Geometry check sheet. Reference: the model listing, model coordinates, mm. A direction names the side the tool comes from. Coordinates: 2 decimals unless noted, no trailing zeros. Order: outer loops, then holes, each group sorted by start corner. A loop starts at its lowest first (then second) coordinate and runs counter-clockwise, first axis right, second up. Notation, with made-up numbers: (48.5, -22) - (101.5, -22) arc R18 cw to (101.5, 13) - close; hole circle Ø4 at (75, -13.5). An arc over 180 degrees is marked (long way). Use CSV: the item, a comma, the result in double quotes. Start each with the question number.
1) Draft check along Z on faces 1 (the flat face through (-4, 0, 5)), 2 (the flat face through (-31, -13, -45.608)), 3 (the cylindrical face through (4.081, -12.522, 50.538)), 4 (the cylindrical face through (-51.136, -12.522, -57.326)). Enter one of: released by +Z, released by -Z, zero draft, split by the parting line, or undercut.
2) Thickness scan on probe 1 along Z at (x, y) = (-35, -23.25); probe 2 along Z at (x, y) = (3.5, -15.25); probe 3 along Z at (x, y) = (-44, -16.5). Record the ranges inside material, lowest first. Write a range as [from, to].
3) Tool access check on faces 5 (the cylindrical face through (-14.022, -12.522, -42.907)), 6 (the flat face through (12.5, -12.5, -29)). Record the directions out of +Z, -Z, +X, -X, +Y, -Y that give a thin tool (end or side, any length) a straight path to the whole face; none if there is none.
4) Sectioned sample at A-A, the plane y = -17.5. Count the separate pieces of the cut face and the enclosed holes in it, and give its area (3 significant figures).
5) Depth check by flat-ended pin: P1, Ø3, axis at y = -22.5, z = -36, coming from the +X side; P2, Ø10, axis at x = -24, z = -19, coming from the -Y side; P3, Ø8, axis at y = -8.5, z = 9, coming from the +X side; P4, Ø12, axis at x = -27.5, y = -10, coming from the -Z side. Enter the tip coordinate at first touch or a pass-through.
6) Sectioned sample at C-C, the plane x = -25. Record the cut outline in (y, z).
7) Sectioned sample at B-B, the plane z = 41. Record the cut outline in (x, y), and give its area (3 significant figures).
from build123d import *

# Parameters (mm, degrees)
F0_R     = 2.8919986146
F1_DEPTH = 25.4


with BuildPart() as f1:
    # F0 (on Front) → F1 (new body)
    with BuildSketch(Plane.XZ):
        with BuildLine():
            ThreePointArc((-15.7877418604, -1.6621768702), (-15.875, -1.428e-07), (-15.7877418904, 1.6621765861))
            Line((-15.7877418904, 1.6621765861), (-15.9627403992, 0))
            Line((-15.9627403992, 0), (-15.7877418604, -1.6621768702))
        make_face()
        with BuildLine():
            ThreePointArc((15.6388934197, -2.7277532162), (15.7630306925, -1.8821499378), (15.8414795915, -1.0310913397))
            Line((15.8414795915, -1.0310913397), (15.6388934197, -2.7277532162))
        make_face()
        with BuildLine():
            ThreePointArc((15.7859080775, 1.6795032503), (15.8527113727, 0.8409323008), (15.875, 0))
            ThreePointArc((15.875, 0), (15.8666176849, -0.515818032), (15.8414795915, -1.0310913397))
            Line((15.8414795915, -1.0310913397), (15.9645947804, 0))
            Line((15.9645947804, 0), (15.7859080775, 1.6795032503))
        make_face()
        with BuildLine():
            ThreePointArc((0, -62.890048396), (6.3233352792, -60.4883240433), (9.4578184155, -54.4943383586))
            ThreePointArc((9.4578184155, -54.4943383586), (9.5081897701, -53.9306916548), (9.525, -53.365048396))
            ThreePointArc((9.525, -53.365048396), (6.7351920908, -46.6298563052), (0, -43.840048396))
            Line((0, -43.840048396), (0, -50.190048396))
            ThreePointArc((0, -50.190048396), (2.2450640303, -51.1199843657), (3.175, -53.365048396))
            ThreePointArc((3.175, -53.365048396), (-0.0112439351, -56.5400284863), (-3.1749203615, -53.3425606669))
            Line((-3.1749203615, -53.3425606669), (-9.5247610846, -53.2975852086))
            ThreePointArc((-9.5247610846, -53.2975852086), (-7.0387492113, -59.7823402345), (-0.8107396043, -62.8554818052))
            Line((-0.8107396043, -62.8554818052), (0, -62.890048396))
        make_face()
        with BuildLine():
            ThreePointArc((-41.6894964213, -45.607795813), (-50.980516261, -57.5603975821), (-36.5115841576, -53.1064395112))
            ThreePointArc((-36.5115841576, -53.1064395112), (-36.5114348356, -53.078330026), (-36.5113850614, -53.0502201884))
            ThreePointArc((-36.5113850614, -53.0502201884), (-37.9332671482, -48.5169399787), (-41.6894964213, -45.607795813))
        make_face()
        with BuildLine():
            ThreePointArc((-41.7578870296, -53.0502201884), (-41.7579039042, -53.0597500804), (-41.7579545278, -53.0692798529))
            ThreePointArc((-41.7579545278, -53.0692798529), (-47.1398662186, -53.0406902964), (-41.7578870296, -53.0502201884))
        make_face(mode=Mode.SUBTRACT)
        with BuildLine():
            ThreePointArc((-15.7877418904, 1.6621765861), (-10.6214069618, 11.7983617147), (0, 15.875))
            Line((0, 15.875), (0, 51.409951604))
            ThreePointArc((0, 51.409951604), (-6.8199440232, 54.2855915957), (-9.5219449967, 61.1761744869))
            Line((-9.5219449967, 61.1761744869), (-15.7877418904, 1.6621765861))
        make_face()
        with BuildLine():
            Line((9.4578184155, -54.4943383586), (15.6388934197, -2.7277532162))
            ThreePointArc((15.6388934197, -2.7277532162), (10.215491733, -12.1515165166), (0, -15.875))
            Line((0, -15.875), (0, -43.840048396))
            ThreePointArc((0, -43.840048396), (6.7351920908, -46.6298563052), (9.525, -53.365048396))
            ThreePointArc((9.525, -53.365048396), (9.5081897701, -53.9306916548), (9.4578184155, -54.4943383586))
        make_face()
        with BuildLine():
            ThreePointArc((0, 51.409951604), (6.6108879801, 54.077708345), (9.5186282495, 60.5866108977))
            ThreePointArc((9.5186282495, 60.5866108977), (9.5234069292, 60.7607521157), (9.525, 60.934951604))
            ThreePointArc((9.525, 60.934951604), (0.1206211137, 70.4591878226), (-9.5219449967, 61.1761744869))
            ThreePointArc((-9.5219449967, 61.1761744869), (-6.8199440232, 54.2855915957), (0, 51.409951604))
        make_face()
        with BuildLine():
            ThreePointArc((3.175, 60.934951604), (2.2450640303, 58.6898875738), (0, 57.759951604))
            ThreePointArc((0, 57.759951604), (-2.2450640303, 63.1800156343), (3.175, 60.934951604))
        make_face(mode=Mode.SUBTRACT)
        with BuildLine():
            Line((0, -50.190048396), (0, -43.840048396))
            ThreePointArc((0, -43.840048396), (-6.7112978678, -46.6060465518), (-9.5247610846, -53.2975852086))
            Line((-9.5247610846, -53.2975852086), (-3.1749203615, -53.3425606669))
            ThreePointArc((-3.1749203615, -53.3425606669), (-2.2370992893, -51.1120477812), (0, -50.190048396))
        make_face()
        with BuildLine():
            ThreePointArc((0, 15.875), (10.6149307794, 11.8041886443), (15.7859080775, 1.6795032503))
            Line((15.7859080775, 1.6795032503), (9.5186282495, 60.5866108977))
            ThreePointArc((9.5186282495, 60.5866108977), (6.6108879801, 54.077708345), (0, 51.409951604))
            Line((0, 51.409951604), (0, 15.875))
        make_face()
        with Locations((4.4577782974, 47.6701632142)):
            Circle(F0_R, mode=Mode.SUBTRACT)
        with BuildLine():
            Line((0, -43.840048396), (0, -15.875))
            ThreePointArc((0, -15.875), (-10.6214068556, -11.7983618103), (-15.7877418604, -1.6621768702))
            Line((-15.7877418604, -1.6621768702), (-12.0856847125, -36.8251776935))
            ThreePointArc((-12.0856847125, -36.8251776935), (-14.0835662669, -42.9767963876), (-19.9921858423, -45.607795813))
            Line((-19.9921858423, -45.607795813), (-41.6894964213, -45.607795813))
            ThreePointArc((-41.6894964213, -45.607795813), (-37.9332671482, -48.5169399787), (-36.5113850614, -53.0502201884))
            ThreePointArc((-36.5113850614, -53.0502201884), (-36.5114348356, -53.078330026), (-36.5115841576, -53.1064395112))
            Line((-36.5115841576, -53.1064395112), (-9.5247610846, -53.2975852086))
            ThreePointArc((-9.5247610846, -53.2975852086), (-6.7112978678, -46.6060465518), (0, -43.840048396))
        make_face()
        with BuildLine():
            Line((0, 3.175), (0, 15.875))
            ThreePointArc((0, 15.875), (-10.6214069618, 11.7983617147), (-15.7877418904, 1.6621765861))
            ThreePointArc((-15.7877418904, 1.6621765861), (-15.875, -1.428e-07), (-15.7877418604, -1.6621768702))
            ThreePointArc((-15.7877418604, -1.6621768702), (-10.6214068556, -11.7983618103), (0, -15.875))
            Line((0, -15.875), (0, -3.175))
            ThreePointArc((0, -3.175), (-3.175, 0), (0, 3.175))
        make_face()
        with BuildLine():
            ThreePointArc((15.8414795915, -1.0310913397), (15.8666176849, -0.515818032), (15.875, 0))
            ThreePointArc((15.875, 0), (15.8527113727, 0.8409323008), (15.7859080775, 1.6795032503))
            ThreePointArc((15.7859080775, 1.6795032503), (10.6149307794, 11.8041886443), (0, 15.875))
            Line((0, 15.875), (0, 3.175))
            ThreePointArc((0, 3.175), (2.2450640303, 2.2450640303), (3.175, 0))
            ThreePointArc((3.175, 0), (2.2450640303, -2.2450640303), (0, -3.175))
            Line((0, -3.175), (0, -15.875))
            ThreePointArc((0, -15.875), (10.215491733, -12.1515165166), (15.6388934197, -2.7277532162))
            Line((15.6388934197, -2.7277532162), (15.8414795915, -1.0310913397))
        make_face()
        with BuildLine():
            ThreePointArc((-0.8107396043, -62.8554818052), (-0.405738079, -62.8814028246), (0, -62.890048396))
            Line((0, -62.890048396), (-0.8107396043, -62.8554818052))
        make_face()
    extrude(amount=F1_DEPTH)


solid = f1.part
Evaluation:
1,face 1,"zero draft"
1,face 2,"released by +Z"
1,face 3,"undercut"
1,face 4,"split by the parting line"
2,probe 1,"[-53.12, -45.61]"
2,probe 2,"[-62.22, 44.94], [50.4, 69.79]"
2,probe 3,"[-60.98, -55.7], [-50.4, -45.13]"
3,face 5,"+Y, -Y"
3,face 6,"-Z, +X, +Y, -Y"
4,separate pieces,"1"
4,enclosed holes,"5"
4,area,"3,500 mm²"
5,P1,"x = 11.85"
5,P2,"through"
5,P3,"x = 15.43"
5,P4,"z = -53.21"
6,outline,"(-25.4, -53.19) - (0, -53.19) - (0, -45.61) - (-25.4, -45.61) - close"
7,outline,"(-11.65, -25.4) - (11.6, -25.4) - (11.6, 0) - (-11.65, 0) - close"
7,area,"591 mm²"
